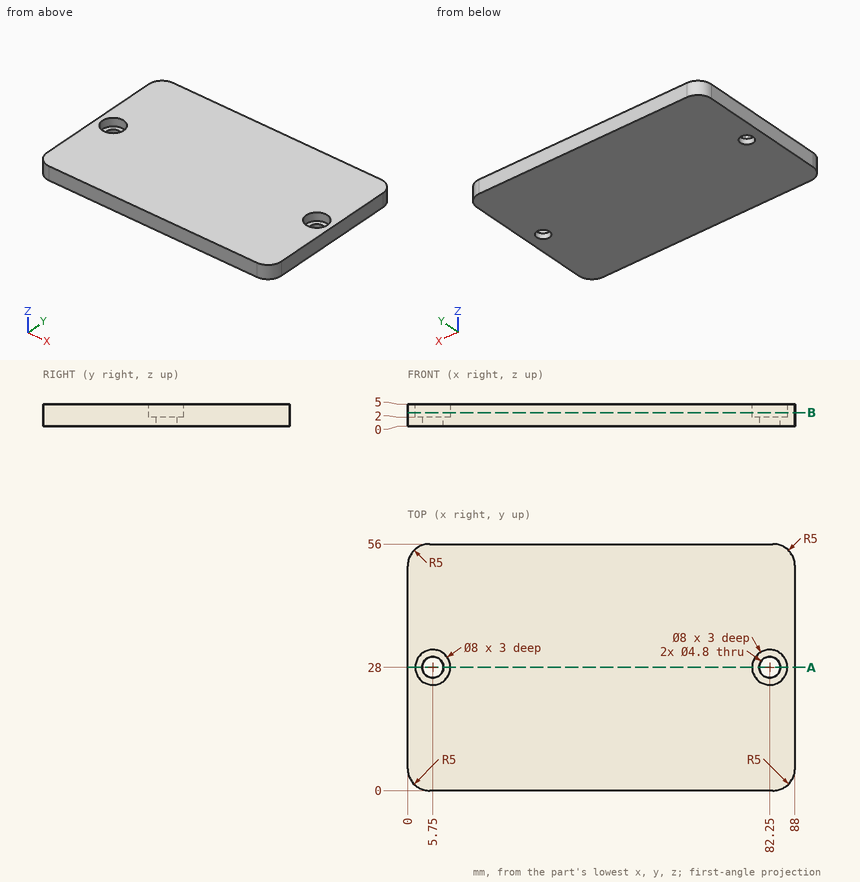
Input: dimensioned drawing with shaded views. Units: mm. Origin: part minimum x, y, z. Give positions to 0.01 mm unless a question says otherwise; leave off trailing zeros. Order: outer loops, then holes, each group sorted by start corner. A loop starts at its lowest first (then second) coordinate and runs counter-clockwise, first axis right, second up. Notation, with made-up numbers: (43, 33) -> (102, 33) arc R10 ccw to (102, 41) -> close; hole circle Ø3 at (60, -33.5). An arc over 180 degrees is marked (long way). Use a Markdown table: item, result.
1) Section query B-B, the plane z = 3.05. Return the cut outline in (x, y).
Answer list:
| item | result |
|---|---|
| outline | (0, 5) arc R5 ccw to (5, 0) -> (83, 0) arc R5 ccw to (88, 5) -> (88, 51) arc R5 ccw to (83, 56) -> (5, 56) arc R5 ccw to (0, 51) -> close; hole circle Ø8 at (5.75, 28); hole circle Ø8 at (82.25, 28) |
2) Contact query for a flat-ended pin moving along its axis: P1, Ø5.5, axis at x = 82.25, y = 28, coming from the +Z side. Output: stop coordinate, or through.
Answer list:
| item | result |
|---|---|
| P1 | z = 2 |
3) Section query A-A, the plane y = 28. Return the cut outline in (x, z).
Answer list:
| item | result |
|---|---|
| outline | (0, 0) -> (3.35, 0) -> (3.35, 2) -> (1.75, 2) -> (1.75, 5) -> (0, 5) -> close; (8.15, 0) -> (79.85, 0) -> (79.85, 2) -> (78.25, 2) -> (78.25, 5) -> (9.75, 5) -> (9.75, 2) -> (8.15, 2) -> close; (84.65, 0) -> (88, 0) -> (88, 5) -> (86.25, 5) -> (86.25, 2) -> (84.65, 2) -> close |
4) Ray query, line 1 along Y through (x, z) = (82.25, 1.15); line 2 along Y through (x, z) = (5.75, 4.4); line 3 along X through (y, z) = (53, 2.95). Return the intervals inside material, ascending. Write a range as [from, to].
Answer list:
| item | result |
|---|---|
| line 1 | [0, 25.6], [30.4, 56] |
| line 2 | [0, 24], [32, 56] |
| line 3 | [0.42, 87.58] |
